```python
from build123d import *

# Parameters (mm, degrees)
SKETCH1_W               = 28.575
SKETCH1_H               = 5.842
SKETCH1_R               = 1.1938
BOSS_EXTRUDE1_DEPTH     = 4.7752
FILLET1_R               = 1.524
CUT_EXTRUDE2_DEPTH      = 16.344948103
CUT_EXTRUDE2_DEPTH_BACK = 16.344948103
SKETCH3_W               = 20.9804
SKETCH3_H               = 2.413


with BuildPart() as part:
    # Sketch1 → Boss-Extrude1 (new body)
    with BuildSketch(Plane(origin=(0, 0, 0), x_dir=(1, 0, 0), z_dir=(0, 1, 0))):
        Rectangle(SKETCH1_W, SKETCH1_H)
        with Locations(Location((12.065, 0, 0), (0, 0, 270))):
            Circle(SKETCH1_R, mode=Mode.SUBTRACT)
        with Locations(Location((-12.065, 0, 0), (0, 0, 270))):
            Circle(SKETCH1_R, mode=Mode.SUBTRACT)
    extrude(amount=BOSS_EXTRUDE1_DEPTH)

    # Fillet1
    fillet1_edges = [part.edges().sort_by_distance(p)[0] for p in [
        (-14.2875, 2.3876, -2.921),
        (14.2875, 2.3876, -2.921),
        (14.2875, 2.3876, 2.921),
        (-14.2875, 2.3876, 2.921),
    ]]
    fillet(fillet1_edges, radius=FILLET1_R)

    # Sketch3 → Cut-Extrude2 (cut, two sides: drawn at the far end of the back side and taken through both)
    with BuildSketch(Plane.XY.offset(-CUT_EXTRUDE2_DEPTH_BACK)):
        with Locations((0, 1.2065)):
            Rectangle(SKETCH3_W, SKETCH3_H)
    extrude(amount=CUT_EXTRUDE2_DEPTH + CUT_EXTRUDE2_DEPTH_BACK, mode=Mode.SUBTRACT)


solid = part.part
```
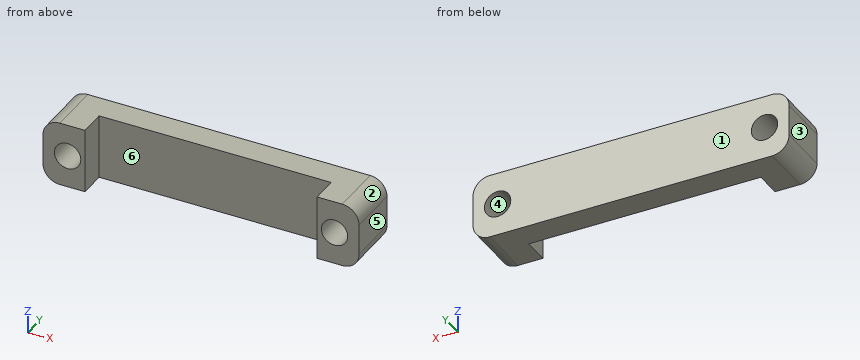
CAD build for the part. Positions are in the model's coordinates, mm. Face numbers are marked on the shaded views. A direction names the side the tool comes from. Round coordinates to 2 decimals unless told otherwise and drop trailing zeros. Order: outer loops, then holes, each group sorted by start corner. A loop starts at its lowest first (then second) coordinate and runs counter-clockwise, first axis right, second up.
Q1. Drop flat-ended pins along their axis: pin 1 (1.5 mm diameter, centred on x = 8.5, y = 1.5, fed in from +Z); pin 2 (1.8 mm diameter, centred on x = 0, z = 1.5, fed in from -Y). Give the stop position or say it passes through.
Q2. Slice it at B-B (x = 11.75). Write the cut outline in (y, z), and give its area (3 significant figures).
Q3. Two-plate mould, pull along X, no slides. Class the marked faces 1, 2, 3 and 4: pulls with the +X half, pulls with the -X half, needs draft (parallel to the pull), parting line crosses it, or undercut.
Q4. Slice it at C-C (y = 1.1). Write the cut outline in (x, z) (1 decimal).
Q5. Slice it at D-D (y = 2.95). Write the cut outline in (x, z) (1 decimal).
Q6. Which spindle directions (+Z, -Z, +X, -X, +Y, -Y) get a long thin tool onto all of the face, cutting with end or side? Do the marked faces 5 and 6. Say none if no direction does.
Q7. Slice it at A-A (z = 0). Write the cut outline in (x, y), and give its area (3 significant figures).
Q8. Wall check: L1, parallel to X at y = 2.35, z = 0; L2, parallel to X at y = 2.8, z = 0; L3, parallel to X at y = 0.4, z = -0.55. Give the ranges that are in metal, low to high.
Results below:
1. pin 1: passes through
1. pin 2: stops at y = 2.41
2. outline: (0, -2.92) - (4.78, -2.92) - (4.78, -1.15) - (0, -1.15) - close; (0, 1.15) - (4.78, 1.15) - (4.78, 2.92) - (0, 2.92) - close
2. area: 16.9 mm2
3. face 1: needs draft
3. face 2: pulls with the +X half
3. face 3: pulls with the -X half
3. face 4: undercut
4. outline: (-14.3, -1.4) arc R1.5 ccw to (-12.8, -2.9) - (-10.5, -2.9) - (-10.5, 2.9) - (-12.8, 2.9) arc R1.5 ccw to (-14.3, 1.4) - close; (10.5, -2.9) - (12.8, -2.9) arc R1.5 ccw to (14.3, -1.4) - (14.3, 1.4) arc R1.5 ccw to (12.8, 2.9) - (10.5, 2.9) - close; hole circle Ø2.4 at (-12.1, 0); hole circle Ø2.4 at (12.1, 0)
5. outline: (-14.3, -1.4) arc R1.5 ccw to (-12.8, -2.9) - (12.8, -2.9) arc R1.5 ccw to (14.3, -1.4) - (14.3, 1.4) arc R1.5 ccw to (12.8, 2.9) - (-12.8, 2.9) arc R1.5 ccw to (-14.3, 1.4) - close; hole circle Ø2.4 at (-12.1, 0); hole circle Ø2.4 at (12.1, 0)
6. face 5: +Z, -Z, +X, +Y, -Y
6. face 6: +Z, -Z, -Y
7. outline: (-14.29, 0) - (-13.26, 0) - (-13.26, 4.78) - (-14.29, 4.78) - close; (-10.87, 0) - (-10.49, 0) - (-10.49, 2.41) - (10.49, 2.41) - (10.49, 0) - (10.87, 0) - (10.87, 4.78) - (-10.87, 4.78) - close; (13.26, 0) - (14.29, 0) - (14.29, 4.78) - (13.26, 4.78) - close
7. area: 63.0 mm2
8. L1: x = -14.29 to -13.26, -10.87 to -10.49, 10.49 to 10.87, 13.26 to 14.29
8. L2: x = -14.29 to -13.26, -10.87 to 10.87, 13.26 to 14.29
8. L3: x = -14.29 to -13.12, -11.01 to -10.49, 10.49 to 11.01, 13.12 to 14.29
